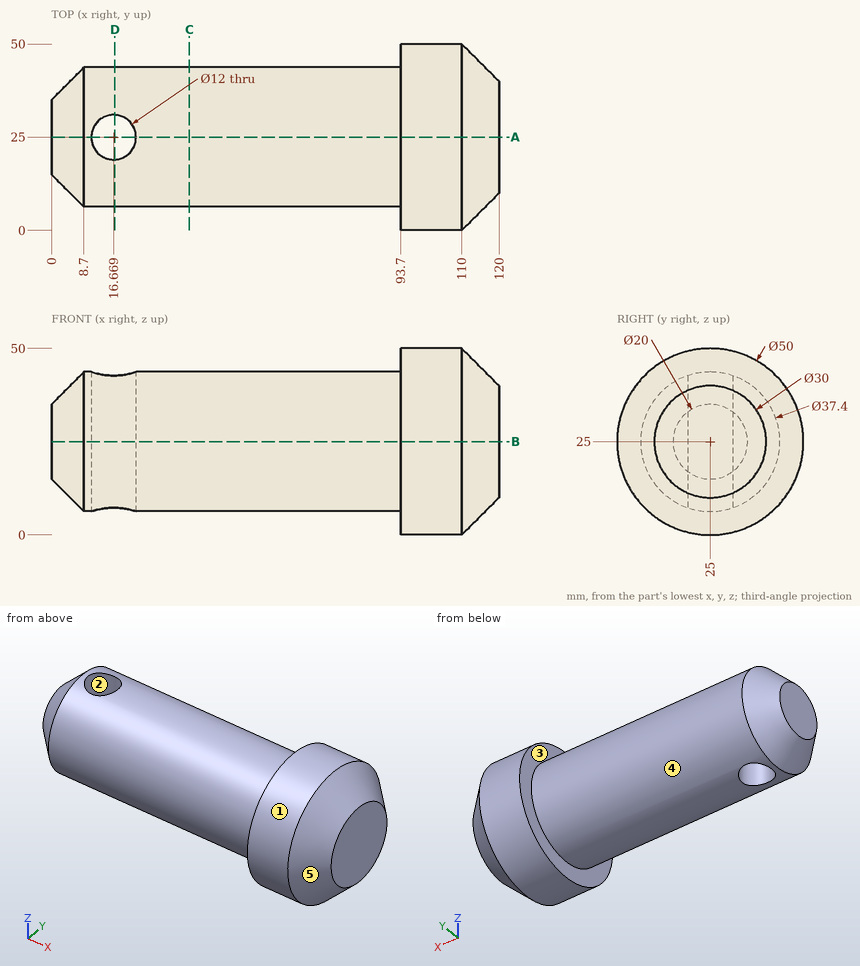
Input: dimensioned drawing with shaded views. Units: mm. Origin: part minimum x, y, z. A direction names the side the tool comes from. Coordinates: 2 decimals unless noted, no trailing zeros. Loops run counter-clockwise (first coordinate to the right, second up) from the corner with the lowest first, then second, coordinate; pieces in that order, holes last. Notation, with made-up numbers: M 6.5,-21 L 36.5,-21 A24 cw 36.5,-9 Z; hole C -16,72 d3. An arc over 180 degrees is marked long. Put each result on its own line as item: value.
(1) Access query for the marked faces 4 and 5. Directions: +Z, -Z, +X, -X, +Y, -Y. A direction counts if a zero-diameter tool reaches every point of the face in a straight line with its end or side. Return the directions, or none.
Answer sheet:
face 4: -X
face 5: +X
(2) Cut plane B-B on z = 25. Return the cut outline in (x, y), then the cut area to 3 significant figures.
Answer sheet:
outline: M 0,15 L 8.7,6.3 L 93.7,6.3 L 93.7,0 L 110,0 L 120,10 L 120,40 L 110,50 L 93.7,50 L 93.7,43.7 L 8.7,43.7 L 0,35 Z; hole C 16.67,25 d12
area: 4,530 mm^2
(3) Cut plane A-A on y = 25. Return the cut outline in (x, z), then the cut area to 4 significant figures.
Answer sheet:
outline: M 0,15 L 8.7,6.3 L 10.67,6.3 L 10.67,43.7 L 8.7,43.7 L 0,35 Z; M 22.67,6.3 L 93.7,6.3 L 93.7,0 L 110,0 L 120,10 L 120,40 L 110,50 L 93.7,50 L 93.7,43.7 L 22.67,43.7 Z
area: 4,195 mm^2
(4) Material intervals for probe 1 along X at (y, z) = (25, 28); probe 2 along X at (y, z) = (22.5, 29.5) (1 decimal); probe 3 along Y at (x, z) = (12.5, 12.5) (1 decimal), sorted ascending.
Answer sheet:
probe 1: x = 0 to 10.67, 22.67 to 120
probe 2: x = 0 to 11.2, 22.1 to 120
probe 3: y = 11.1 to 20.7, 29.3 to 38.9
(5) Draft query along Y for the marked faces 1, 2 and 3. Return one class per face: pulls with the +Y half, pulls with the -Y half, needs draft (parallel to the pull), parting line crosses it, or undercut.
Answer sheet:
face 1: parting line crosses it
face 2: undercut
face 3: needs draft
(6) First-contact query: pin 1 (9.5 mm diameter, centred on x = 16.67, y = 25, fed in from -Z); pin 2 (12 mm diameter, centred on x = 102, z = 38, fed in from +Y); pin 3 (12 mm diameter, centred on x = 40, y = 26, fed in from +Z); pin 4 (1.5 mm diameter, centred on y = 6, z = 17.5, fed in from +X). Flat tips, straight axial feed; report the tip coordinate or a pass-through.
Answer sheet:
pin 1: passes through
pin 2: stops at y = 49
pin 3: stops at z = 43.7
pin 4: stops at x = 115.32
(7) Cut plane D-D on x = 17. Return the cut outline in (y, z) (1 decimal).
Answer sheet:
outline: M 19,7.3 L 19,42.7 A18.7 ccw Z; M 31,7.3 A18.7 ccw 31,42.7 Z
(8) Cut plane C-C on x = 37. Return the cut outline in (y, z), then the cut area to 3 significant figures.
Answer sheet:
outline: C 25,25 d37.4
area: 1,100 mm^2
